from build123d import *

# Parameters (mm, degrees)
SKETCH2_W           = 0.63000001
SKETCH2_H           = 6
BOSS_EXTRUDE1_DEPTH = 50.8


with BuildPart() as part:
    # Sweep1: sweep along a path in Sketch1
    with BuildLine(Plane(origin=(0, 0, 0), x_dir=(1, 0, 0), z_dir=(0, 1, 0))) as sweep1_path:
        Line((-18.8468, -25.4), (-18.8468, 0))
        ThreePointArc((-18.8468, 0), (0.164467269, 18.846082372), (18.843929541, -0.328922014))
        Line((18.843929541, -0.328922014), (16.1841828, -152.705710755))
    # Sketch2 → Sweep1 (sweep)
    with BuildSketch(Plane(origin=(-18.8468, 0, 25.4), x_dir=(-1, 0, 0), z_dir=(0, 0, -1))):
        with Locations((0.315000005, -3)):
            Rectangle(SKETCH2_W, SKETCH2_H)
    sweep(path=sweep1_path.line)

    # Sketch3 → Boss-Extrude1 (add)
    with BuildSketch(Plane.XY.offset(25.4)):
        Polygon((-21.060381709, -0.655941017), (-16.817741022, -4.898581704), (-17.263218301, -5.344058983), (-21.505858988, -1.101418296), align=None)
    extrude(amount=BOSS_EXTRUDE1_DEPTH)


solid = part.part
Work out the finished part from the listing and answer in its coordinate system (mm). A direction names the side the tool comes from. Round coordinates to 2 decimals unless told otherwise and drop trailing zeros. Write each loop counter-clockwise with the first axis right and the second up, starting at its lowest first coordinate (ties: lowest second). Pieces come first, ordered by that corner, then holes. Notation, with made-up numbers: (66, 76) - (91, 76) arc R6 ccw to (91, 80) - close; hole circle Ø4 at (54.5, 78). An arc over 180 degrees is marked (long way). Answer in a Markdown table with one row per item. Add a question column.
1. Given pin 1 (2 mm diameter, centred on y = -4.5, z = 116.5, fed in from -X); pin 2 (0.6 mm diameter, centred on x = -20.5, y = -1.5, fed in from -Z); pin 3 (0.6 mm diameter, centred on x = -18, y = -4, fed in from -Z), each flat-ended and moving along its own axis, determine where each tip first touches the part or whether it passes through.
2. The mould has two halves that part along X. Classify faces 4 (the flat face through (-18.847, -3, 13)), 5 (the cylindrical face through (-0.261, -2.958, -19.475)), 6 (the flat face through (-19.355, -3.252, 50.444)): +X half, -X half, draft (parallel to the pull), parting line (faces both ways), or undercut.
3. A cutting plane is placed at A-A, the plane z = -3. Determine the outline of the cut face in (x, y).
4. A cutting plane is placed at B-B, the plane x = 0. Determine the outline of the cut face in (y, z), and give its area (3 significant figures).
5. Find the intervals of material crossed by line 1 along X through (y, z) = (-0.9, 0); line 2 along X through (y, z) = (-1.15, -11); line 3 along Z through (x, y) = (10.5, -2.9), in increasing order. Write a range as from..to.
6. A cutting plane is placed at C-C, the plane z = 27. Determine the outline of the cut face in (x, y), and give its area (3 significant figures).
7. For faces 1 (the flat face through (-19, -3, 76.2)), 2 (the cylindrical face through (-0.252, -3.042, -18.845)), 3 (the flat face through (-18.969, -2.748, 50.444)), determine the directions among +Z, -Z, +X, -X, +Y, -Y from which every point of the face is accessible in a straight line to the end or side of a thin tool.
8. A cutting plane is placed at D-D, the plane z = 95. Determine the outline of the cut face in (x, y), and give its area (3 significant figures).
Worked out:
| question | item | result |
|---|---|---|
| 1 | pin 1 | x = 16.8 |
| 1 | pin 2 | z = 25.4 |
| 1 | pin 3 | z = -8.13 |
| 2 | face 4 | undercut |
| 2 | face 5 | parting line |
| 2 | face 6 | -X half |
| 3 | outline | (-19.24, -6) - (-18.61, -6) - (-18.61, 0) - (-19.24, 0) - close; (18.61, -6) - (19.24, -6) - (19.24, 0) - (18.61, 0) - close |
| 4 | outline | (-6, -19.48) - (0, -19.48) - (0, -18.85) - (-6, -18.85) - close |
| 4 | area | 3.78 mm^2 |
| 5 | line 1 | -19.48..-18.85, 18.85..19.48 |
| 5 | line 2 | -16.07..-15.3, 15.3..16.07 |
| 5 | line 3 | -16.4..-15.65 |
| 6 | outline | (-21.51, -1.1) - (-17.26, -5.34) - (-16.82, -4.9) - (-21.06, -0.66) - close; (18.38, -6) - (19.01, -6) - (19.01, 0) - (18.38, 0) - close |
| 6 | area | 7.56 mm^2 |
| 7 | face 1 | +Z, -X, +Y, -Y |
| 7 | face 2 | +Y, -Y |
| 7 | face 3 | +Z, +Y |
| 8 | outline | (17.19, -6) - (17.82, -6) - (17.82, 0) - (17.19, 0) - close |
| 8 | area | 3.78 mm^2 |
